from build123d import *

# Parameters (mm, degrees)
CYLINDER001_R     = 22.5
CYLINDER001_DEPTH = 10
CYLINDER017_R     = 4
CYLINDER017_DEPTH = 22.5
CYLINDER016_R     = 4
CYLINDER016_DEPTH = 22.5
CYLINDER015_R     = 4
CYLINDER015_DEPTH = 28.5
CYLINDER013_R     = 2.25
CYLINDER013_DEPTH = 65
CYLINDER012_R     = 2.25
CYLINDER012_DEPTH = 65
PAD004_DEPTH      = 4
PAD003_DEPTH      = 4
CYLINDER014_R     = 4
CYLINDER014_DEPTH = 28.5
BOX002_W          = 65
BOX002_H          = 10
BOX002_DEPTH      = 27.5
FILLET001_R       = 4


with BuildPart() as cylinder001:
    # Cylinder001 → Cylinder001 (new body)
    with BuildSketch(Plane(origin=(0, 10, 37.5), x_dir=(1, 0, 0), z_dir=(0, -1, 0))):
        Circle(CYLINDER001_R)
    extrude(amount=CYLINDER001_DEPTH)


with BuildPart() as cylinder017:
    # Cylinder017 → Cylinder017 (new body)
    with BuildSketch(Plane(origin=(-27.5, 5, 0), x_dir=(1, 0, 0), z_dir=(0, 0, 1))):
        Circle(CYLINDER017_R)
    extrude(amount=CYLINDER017_DEPTH)


with BuildPart() as fusion009:
    # Cylinder016 → Cylinder016 (new body)
    with BuildSketch(Plane(origin=(27.5, 5, 0), x_dir=(1, 0, 0), z_dir=(0, 0, 1))):
        Circle(CYLINDER016_R)
    extrude(amount=CYLINDER016_DEPTH)

    # Fusion009: union Cylinder017
    add(cylinder017.part)


with BuildPart() as fusion009_1:
    # Fusion009 placement: moved
    add(fusion009.part.moved(Location((0, 0, 42.5))))


with BuildPart() as cylinder015:
    # Cylinder015 → Cylinder015 (new body)
    with BuildSketch(Plane(origin=(-27.5, 5, 0), x_dir=(1, 0, 0), z_dir=(0, 0, 1))):
        Circle(CYLINDER015_R)
    extrude(amount=CYLINDER015_DEPTH)


with BuildPart() as cylinder013:
    # Cylinder013 → Cylinder013 (new body)
    with BuildSketch(Plane(origin=(-27.5, 5, 0), x_dir=(1, 0, 0), z_dir=(0, 0, 1))):
        Circle(CYLINDER013_R)
    extrude(amount=CYLINDER013_DEPTH)


with BuildPart() as fusion007:
    # Cylinder012 → Cylinder012 (new body)
    with BuildSketch(Plane(origin=(27.5, 5, 0), x_dir=(1, 0, 0), z_dir=(0, 0, 1))):
        Circle(CYLINDER012_R)
    extrude(amount=CYLINDER012_DEPTH)

    # Fusion007: union Cylinder013
    add(cylinder013.part)


with BuildPart() as m4press003:
    # Sketch004 → Pad004 (new body)
    with BuildSketch(Plane.XY):
        Polygon((4, 0), (2, 3.464102), (-2, 3.464102), (-4, 0), (-2, -3.464102), (2, -3.464102), align=None)
    extrude(amount=PAD004_DEPTH)


with BuildPart() as m4press003_1:
    # Body004 placement: moved
    add(m4press003.part.moved(Location((27.5, 5, 28.5))))


with BuildPart() as m4press002:
    # Sketch003 → Pad003 (new body)
    with BuildSketch(Plane.XY):
        Polygon((4, 0), (2, 3.464102), (-2, 3.464102), (-4, 0), (-2, -3.464102), (2, -3.464102), align=None)
    extrude(amount=PAD003_DEPTH)


with BuildPart() as m4press002_1:
    # Body003 placement: moved
    add(m4press002.part.moved(Location((-27.5, 5, 28.5))))


with BuildPart() as connectors001:
    # Cylinder014 → Cylinder014 (new body)
    with BuildSketch(Plane(origin=(27.5, 5, 0), x_dir=(1, 0, 0), z_dir=(0, 0, 1))):
        Circle(CYLINDER014_R)
    extrude(amount=CYLINDER014_DEPTH)

    # Fusion008: union Cylinder015, Fusion007, M4Press003, M4Press002
    add(cylinder015.part)
    add(fusion007.part)
    add(m4press003_1.part)
    add(m4press002_1.part)


with BuildPart() as upper_part:
    # Box002 → Box002 (new body)
    with BuildSketch(Plane(origin=(-32.5, 0, 37.5), x_dir=(1, 0, 0), z_dir=(0, 0, 1))):
        with Locations((32.5, 5)):
            Rectangle(BOX002_W, BOX002_H)
    extrude(amount=BOX002_DEPTH)

    # Cut003: cut Connectors001
    add(connectors001.part, mode=Mode.SUBTRACT)

    # Cut004: cut Fusion009
    add(fusion009_1.part, mode=Mode.SUBTRACT)

    # Cut005: cut Cylinder001
    add(cylinder001.part, mode=Mode.SUBTRACT)

    # Fillet001
    fillet001_edges = [upper_part.edges().sort_by_distance(p)[0] for p in [
        (-32.5, 5, 65),
        (32.5, 5, 65),
    ]]
    fillet(fillet001_edges, radius=FILLET001_R)


solid = upper_part.part
Geometry: final body of the model. Coordinates: model frame, mm. A direction names the side the tool comes from. Coordinates: 2 decimals unless noted, no trailing zeros. Loops run counter-clockwise (first coordinate to the right, second up) from the corner with the lowest first, then second, coordinate; pieces in that order, holes last. Notation, with made-up numbers: M 46,59.25 L 96,59.25 A29 cw 96,90.25 Z; hole C 83.5,64.25 d7. An arc over 180 degrees is marked long. One line per item, written item: value. Start each with the question number.
1) Cut plane C-C (z = 56.5). Return loops of the section in (x, y), then the cut area to 3 significant figures.
2) Reachability of faces 1 (the flat face through (29, 3, 42.5)), 2 (the cylindrical face through (31.297, 0.571, 63.859)), 3 (the cylindrical face through (31.297, 9.444, 63.859)), 4 (the cylindrical face through (-31.359, 9.444, 63.797)), 5 (the cylindrical face through (-31.359, 0.571, 63.797)) from +Z, -Z, +X, -X, +Y, -Y: full face, straight path, thin tool, end or side. Return the list, or none.
3) Material intervals for L1, parallel to Y at x = 27.5, z = 59.75; L2, parallel to X at y = 8.25, z = 50; L3, parallel to X at y = 5, z = 56.25, sorted ascending. Write a range as from..to.
4) Pin query (flat end, axial travel): P1, Ø6, axis at x = 27.5, y = 5, coming from the -Z side; P2, Ø1, axis at x = 6.5, y = 6.5, coming from the -Z side; P3, Ø1.5, axis at x = -6.5, y = 6, coming from the -Z side; P4, Ø4, axis at x = 28, y = 4.5, coming from the +Z side. Return the tip coordinate at first contact, or that it passes through.
5) Cut plane A-A (x = 27.5). Return loops of the section in (y, z).
6) Cut plane D-D (x = 0). Return loops of the section in (y, z).
7) Cut plane B-B (z = 47.5). Return loops of the section in (x, y).
8) Draft query along Y for faces 6 (the cylindrical face through (29.646, 5.676, 39.965)), 7 (the flat face through (-30, 5, 37.5)), 8 (the flat face through (-0.5, 0, 60.2)), 9 (the flat face through (-0.5, 10, 60.2)). Return one class per face: released by +Y, released by -Y, zero draft, split by the parting line, or undercut.
Evaluation:
1. outline: M -32.5,0 L -12.05,0 L -12.05,10 L -32.5,10 Z; M 12.05,0 L 32.5,0 L 32.5,10 L 12.05,10 Z; hole C -27.5,5 d8; hole C 27.5,5 d8
1. area: 308 mm^2
2. face 1: +Z
2. face 2: +Z, +X, -Y
2. face 3: +Z, +X, +Y
2. face 4: +Z, -X, +Y
2. face 5: +Z, -X, -Y
3. L1: 0..1, 9..10
3. L2: -32.5..-29.83, -25.17..-18.71, 18.71..25.17, 29.83..32.5
3. L3: -32.5..-31.5, -23.5..-12.44, 12.44..23.5, 31.5..32.5
4. P1: z = 37.5
4. P2: z = 58.88
4. P3: z = 58.8
4. P4: z = 42.5
5. outline: M 0,37.5 L 2.75,37.5 L 2.75,42.5 L 1,42.5 L 1,65 L 0,65 Z; M 7.25,37.5 L 10,37.5 L 10,65 L 9,65 L 9,42.5 L 7.25,42.5 Z
6. outline: M 0,60 L 10,60 L 10,65 L 0,65 Z
7. outline: M -32.5,0 L -20.16,0 L -20.16,10 L -32.5,10 Z; M 20.16,0 L 32.5,0 L 32.5,10 L 20.16,10 Z; hole C -27.5,5 d8; hole C 27.5,5 d8
8. face 6: undercut
8. face 7: zero draft
8. face 8: released by -Y
8. face 9: released by +Y
